```python
from build123d import *

# Parameters (mm, degrees)
SKETCH_1_R          = 6.5
EXTRUDE_1_DEPTH     = 1
EXTRUDE_2_DEPTH     = 5.5
EXTRUDE_3_DEPTH     = 1.1
SKETCH_5_R          = 4
CUT_EXTRUDE_1_DEPTH = 7.5
SKETCH_6_R          = 5.11
CUT_EXTRUDE_2_DEPTH = 0.2


with BuildPart() as part:
    # 草图1 → 拉伸1 (new body)
    with BuildSketch(Plane.XY):
        Circle(SKETCH_1_R)
    extrude(amount=EXTRUDE_1_DEPTH)

    # 草图2 → 拉伸2 (add)
    with BuildSketch(Plane.XY.offset(1)):
        Polygon((0, 9.192388155), (-9.192388155, 0), (0, -9.192388155), (9.192388155, 0), align=None)
    extrude(amount=EXTRUDE_2_DEPTH)

    # 草图3 → 拉伸3 (add)
    with BuildSketch(Plane.XY.offset(6.5)):
        Polygon((9.192388155, 0), (0, 9.192388155), (-9.192388155, 0), (0, -9.192388155), align=None)
    extrude(amount=EXTRUDE_3_DEPTH)

    # 草图4 → 切除-旋转1 (revolve, cut)
    with BuildSketch(Plane(origin=(0, 0, 0), x_dir=(0, 0, -1), z_dir=(1, 0, 0))):
        Polygon((-6.5, 6.592388155), (-6.5, 0), (-7.6, 0), (-7.6, 7.692388155), align=None)
    revolve(axis=Axis((0, 0, 0), (0, 0, 1)), mode=Mode.SUBTRACT)

    # 草图5 → 切除-拉伸1 (cut, through all)
    with BuildSketch(Plane.XY.offset(6.5)):
        Circle(SKETCH_5_R)
    extrude(amount=-CUT_EXTRUDE_1_DEPTH, mode=Mode.SUBTRACT)

    # 草图6 → 切除-拉伸2 (cut)
    with BuildSketch(Plane(origin=(0, 0, 0), x_dir=(-1, 0, 0), z_dir=(0, 0, -1))):
        Circle(SKETCH_6_R)
    extrude(amount=-CUT_EXTRUDE_2_DEPTH, mode=Mode.SUBTRACT)


solid = part.part
```
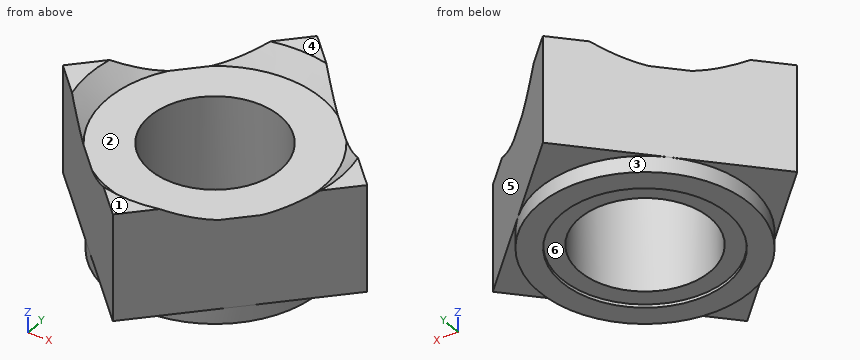
Source: CAD feature listing. Evaluate the final solid. Frame: model axes, mm. Face numbers are marked on the shaded views. A direction names the side the tool comes from. Round coordinates to 2 decimals unless told otherwise and drop trailing zeros. Loops run counter-clockwise (first coordinate to the right, second up) from the corner with the lowest first, then second, coordinate; pieces in that order, holes last.
1. Contact query for flat-ended pins moving along their axis: pin 1 (4 mm diameter, centred on x = 5, z = 4, fed in from +Y); pin 2 (1.4 mm diameter, centred on x = 7.5, y = -0.5, fed in from -Z); pin 3 (3 mm diameter, centred on y = -2, z = 2.5, fed in from +X). Output: stop coordinate, or through.
2. Section query A-A on z = 2.5. Output: boundary loops of the cut face in (x, y).
3. Ray query, L1, parallel to Y at x = 0, z = 0.15; L2, parallel to Z at x = 3, y = 3.5; L3, parallel to X at y = -0.5, z = 1.5. Return the intervals inside material, ascending.
4. Access query for the marked faces 1, 2 and 3. Directions: +Z, -Z, +X, -X, +Y, -Y. A direction counts if a zero-diameter tool reaches every point of the face in a straight line with its end or side. Return the directions, or none.
5. Mould query, pull axis X, two halves, no side actions, for the marked faces 4, 5 and 6. Classes: released by +X, released by -X, zero draft, split by the parting line, or undercut.
Answers below:
1. pin 1: stops at y = 6.19
1. pin 2: stops at z = 1
1. pin 3: stops at x = 8.69
2. outline: (-9.19, 0) - (0, -9.19) - (9.19, 0) - (0, 9.19) - close; hole circle Ø8 at (0, 0)
3. L1: y = -6.5 to -5.11, 5.11 to 6.5
3. L2: z = 0.2 to 6.5
3. L3: x = -8.69 to -3.97, 3.97 to 8.69
4. face 1: +Z, +X, -X, +Y, -Y
4. face 2: +Z
4. face 3: -Z
5. face 4: zero draft
5. face 5: released by +X
5. face 6: undercut
